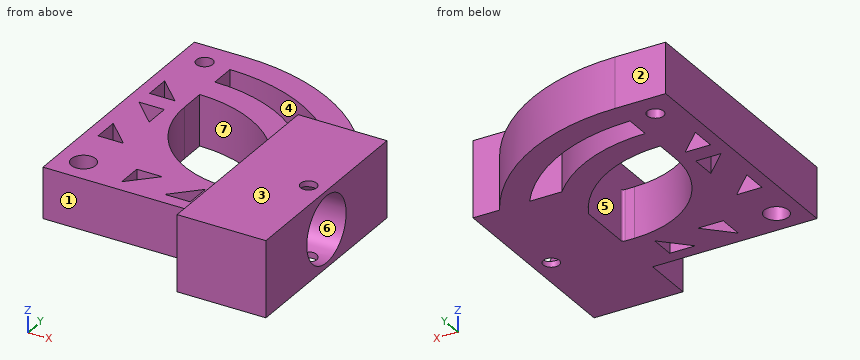
from build123d import *

# Parameters (mm, degrees)
F0_R     = 4.75
F1_DEPTH = 20
F2_DEPTH = 30
F3_R     = 13
F4_DEPTH = 25


with BuildPart() as f1:
    # F0 (on Top) → F1 (new body)
    with BuildSketch(Plane.XY):
        with BuildLine():
            Line((76.6160202911, 30.1966461055), (66.1766930438, 30.1966461055))
            ThreePointArc((66.1766930438, 30.1966461055), (73.2373422542, 14.1088810364), (76.6160202911, -3.132159736))
            Line((76.6160202911, -3.132159736), (76.6160202911, 30.1966461055))
        make_face()
        with BuildLine():
            ThreePointArc((76.6160202911, -3.132159736), (73.2373422542, 14.1088810364), (66.1766930438, 30.1966461055))
            Line((66.1766930438, 30.1966461055), (54.3402872065, 30.1966461055))
            ThreePointArc((54.3402872065, 30.1966461055), (63.4377209443, 11.9226935784), (66.8762698088, -8.198862606))
            ThreePointArc((66.8762698088, -8.198862606), (70.4472594921, -6.7390976404), (72.7910202911, -9.8033538945))
            ThreePointArc((72.7910202911, -9.8033538945), (70.4472594921, -12.8676101486), (66.8762698088, -11.407845183))
            ThreePointArc((66.8762698088, -11.407845183), (63.4377209443, -31.5294013674), (54.3402872065, -49.8033538945))
            Line((54.3402872065, -49.8033538945), (66.1766930438, -49.8033538945))
            ThreePointArc((66.1766930438, -49.8033538945), (73.2373422542, -33.7155888254), (76.6160202911, -16.474548053))
            Line((76.6160202911, -16.474548053), (76.6160202911, -3.132159736))
        make_face()
        with BuildLine():
            ThreePointArc((66.8762698088, -8.198862606), (63.4377209443, 11.9226935784), (54.3402872065, 30.1966461055))
            Line((54.3402872065, 30.1966461055), (41.6160202911, 30.1966461055))
            ThreePointArc((41.6160202911, 30.1966461055), (52.9450022789, 11.6059714919), (56.8946607411, -9.8033538945))
            ThreePointArc((56.8946607411, -9.8033538945), (52.9450022789, -31.2126792809), (41.6160202911, -49.8033538945))
            Line((41.6160202911, -49.8033538945), (54.3402872065, -49.8033538945))
            ThreePointArc((54.3402872065, -49.8033538945), (63.4377209443, -31.5294013674), (66.8762698088, -11.407845183))
            ThreePointArc((66.8762698088, -11.407845183), (66.4410202911, -9.8033538945), (66.8762698088, -8.198862606))
        make_face()
        with BuildLine():
            ThreePointArc((76.6160202911, -16.474548053), (73.2373422542, -33.7155888254), (66.1766930438, -49.8033538945))
            Line((66.1766930438, -49.8033538945), (76.6160202911, -49.8033538945))
            Line((76.6160202911, -49.8033538945), (76.6160202911, -16.474548053))
        make_face()
        with BuildLine():
            ThreePointArc((56.8946607411, -9.8033538945), (52.9450022789, 11.6059714919), (41.6160202911, 30.1966461055))
            Line((41.6160202911, 30.1966461055), (41.6160202911, 12.5573258805))
            ThreePointArc((41.6160202911, 12.5573258805), (45.5571102145, 1.6842921329), (46.8946607411, -9.8033538945))
            ThreePointArc((46.8946607411, -9.8033538945), (45.5571102145, -21.2909999219), (41.6160202911, -32.1640336695))
            Line((41.6160202911, -32.1640336695), (41.6160202911, -49.8033538945))
            ThreePointArc((41.6160202911, -49.8033538945), (52.9450022789, -31.2126792809), (56.8946607411, -9.8033538945))
        make_face()
        with BuildLine():
            ThreePointArc((46.8946607411, -9.8033538945), (45.5571102145, 1.6842921329), (41.6160202911, 12.5573258805))
            Line((41.6160202911, 12.5573258805), (41.6160202911, -8.8033538945))
            Line((41.6160202911, -8.8033538945), (41.6160202911, -29.8033538945))
            Line((41.6160202911, -29.8033538945), (41.6160202911, -30.8033538945))
            Line((41.6160202911, -30.8033538945), (41.6160202911, -32.1640336695))
            ThreePointArc((41.6160202911, -32.1640336695), (45.5571102145, -21.2909999219), (46.8946607411, -9.8033538945))
        make_face()
        with BuildLine():
            Line((-3.1053392589, 30.1966461055), (-3.1053392589, 40.1966461055))
            ThreePointArc((-3.1053392589, 40.1966461055), (-8.9600600243, 39.8526854639), (-14.7342290493, 38.8255358959))
            Line((-14.7342290493, 38.8255358959), (-8.1053392589, 32.1966461055))
            Line((-8.1053392589, 32.1966461055), (-18.1053392589, 32.1966461055))
            Line((-18.1053392589, 32.1966461055), (-18.1053392589, 37.8936061763))
            ThreePointArc((-18.1053392589, 37.8936061763), (-20.630331421, 37.0247856128), (-23.1053392589, 36.0224030551))
            Line((-23.1053392589, 36.0224030551), (-23.1053392589, -29.8033538945))
            Line((-23.1053392589, -29.8033538945), (-3.1053392589, -29.8033538945))
            Line((-3.1053392589, -29.8033538945), (40.6160202911, -29.8033538945))
            Line((40.6160202911, -29.8033538945), (41.6160202911, -29.8033538945))
            Line((41.6160202911, -29.8033538945), (41.6160202911, -8.8033538945))
            ThreePointArc((41.6160202911, -8.8033538945), (41.3231270723, -9.5104606757), (40.6160202911, -9.8033538945))
            Line((40.6160202911, -9.8033538945), (36.8946607411, -9.8033538945))
            ThreePointArc((36.8946607411, -9.8033538945), (8.6103894936, 1.912374858), (-3.1053392589, 30.1966461055))
        make_face()
        with Locations((-13.1053392589, -19.8033538945)):
            Circle(F0_R, mode=Mode.SUBTRACT)
        Polygon((4.8946607411, -14.8033538945), (14.8946607411, -14.8033538945), (4.8946607411, -24.8033538945), align=None, mode=Mode.SUBTRACT)
        Polygon((31.8946607411, -24.8033538945), (21.8946607411, -24.8033538945), (31.8946607411, -14.8033538945), align=None, mode=Mode.SUBTRACT)
        Polygon((-18.1053392589, -1.8033538945), (-18.1053392589, 8.1966461055), (-8.1053392589, -1.8033538945), align=None, mode=Mode.SUBTRACT)
        Polygon((-8.1053392589, 25.1966461055), (-8.1053392589, 15.1966461055), (-18.1053392589, 25.1966461055), align=None, mode=Mode.SUBTRACT)
        with BuildLine():
            Line((-3.1053392589, 40.1966461055), (-3.1053392589, 50.1966461055))
            ThreePointArc((-3.1053392589, 50.1966461055), (-13.2514579825, 49.3325596847), (-23.1053392589, 46.7651886004))
            Line((-23.1053392589, 46.7651886004), (-23.1053392589, 36.0224030551))
            ThreePointArc((-23.1053392589, 36.0224030551), (-20.630331421, 37.0247856128), (-18.1053392589, 37.8936061763))
            Line((-18.1053392589, 37.8936061763), (-18.1053392589, 42.1966461055))
            Line((-18.1053392589, 42.1966461055), (-14.7342290493, 38.8255358959))
            ThreePointArc((-14.7342290493, 38.8255358959), (-8.9600600243, 39.8526854639), (-3.1053392589, 40.1966461055))
        make_face()
        with BuildLine():
            Line((-3.1053392589, 50.1966461055), (-3.1053392589, 60.1966461055))
            ThreePointArc((-3.1053392589, 60.1966461055), (-6.4925947199, 60.1146445068), (-9.8719141705, 59.8688318324))
            ThreePointArc((-9.8719141705, 59.8688318324), (-12.6457198511, 56.9793102511), (-16.1176393473, 58.9765853786))
            ThreePointArc((-16.1176393473, 58.9765853786), (-19.6333066276, 58.2174245093), (-23.1053392589, 57.2786854305))
            Line((-23.1053392589, 57.2786854305), (-23.1053392589, 46.7651886004))
            ThreePointArc((-23.1053392589, 46.7651886004), (-13.2514579825, 49.3325596847), (-3.1053392589, 50.1966461055))
        make_face()
        with BuildLine():
            Line((-3.1053392589, 60.1966461055), (-3.1053392589, 70.1966461055))
            ThreePointArc((-3.1053392589, 70.1966461055), (-13.1856826575, 69.5590218069), (-23.1053392589, 67.6563130296))
            Line((-23.1053392589, 67.6563130296), (-23.1053392589, 57.2786854305))
            ThreePointArc((-23.1053392589, 57.2786854305), (-19.6333066276, 58.2174245093), (-16.1176393473, 58.9765853786))
            ThreePointArc((-16.1176393473, 58.9765853786), (-13.7268393445, 63.3866676797), (-9.8553392589, 60.1966461055))
            ThreePointArc((-9.8553392589, 60.1966461055), (-9.8594856318, 60.0325295879), (-9.8719141705, 59.8688318324))
            ThreePointArc((-9.8719141705, 59.8688318324), (-6.4925947199, 60.1146445068), (-3.1053392589, 60.1966461055))
        make_face()
        with BuildLine():
            ThreePointArc((-23.1053392589, 67.6563130296), (-13.1856826575, 69.5590218069), (-3.1053392589, 70.1966461055))
            Line((-3.1053392589, 70.1966461055), (-23.1053392589, 70.1966461055))
            Line((-23.1053392589, 70.1966461055), (-23.1053392589, 67.6563130296))
        make_face()
        with BuildLine():
            ThreePointArc((66.1766930438, 30.1966461055), (36.8946607411, 59.4786784083), (-3.1053392589, 70.1966461055))
            Line((-3.1053392589, 70.1966461055), (-3.1053392589, 60.1966461055))
            ThreePointArc((-3.1053392589, 60.1966461055), (29.2983642331, 52.2450143355), (54.3402872065, 30.1966461055))
            Line((54.3402872065, 30.1966461055), (66.1766930438, 30.1966461055))
        make_face()
        with BuildLine():
            ThreePointArc((41.6160202911, 30.1966461055), (21.3895581689, 44.968901856), (-3.1053392589, 50.1966461055))
            Line((-3.1053392589, 50.1966461055), (-3.1053392589, 40.1966461055))
            ThreePointArc((-3.1053392589, 40.1966461055), (23.181216347, 32.7291865231), (41.6160202911, 12.5573258805))
            Line((41.6160202911, 12.5573258805), (41.6160202911, 30.1966461055))
        make_face()
    extrude(amount=F1_DEPTH)

    # F0 (on Top) → F2 (join)
    with BuildSketch(Plane.XY):
        with BuildLine():
            ThreePointArc((56.8946607411, -9.8033538945), (52.9450022789, 11.6059714919), (41.6160202911, 30.1966461055))
            Line((41.6160202911, 30.1966461055), (41.6160202911, 12.5573258805))
            ThreePointArc((41.6160202911, 12.5573258805), (45.5571102145, 1.6842921329), (46.8946607411, -9.8033538945))
            ThreePointArc((46.8946607411, -9.8033538945), (45.5571102145, -21.2909999219), (41.6160202911, -32.1640336695))
            Line((41.6160202911, -32.1640336695), (41.6160202911, -49.8033538945))
            ThreePointArc((41.6160202911, -49.8033538945), (52.9450022789, -31.2126792809), (56.8946607411, -9.8033538945))
        make_face()
        with BuildLine():
            ThreePointArc((66.8762698088, -8.198862606), (63.4377209443, 11.9226935784), (54.3402872065, 30.1966461055))
            Line((54.3402872065, 30.1966461055), (41.6160202911, 30.1966461055))
            ThreePointArc((41.6160202911, 30.1966461055), (52.9450022789, 11.6059714919), (56.8946607411, -9.8033538945))
            ThreePointArc((56.8946607411, -9.8033538945), (52.9450022789, -31.2126792809), (41.6160202911, -49.8033538945))
            Line((41.6160202911, -49.8033538945), (54.3402872065, -49.8033538945))
            ThreePointArc((54.3402872065, -49.8033538945), (63.4377209443, -31.5294013674), (66.8762698088, -11.407845183))
            ThreePointArc((66.8762698088, -11.407845183), (66.4410202911, -9.8033538945), (66.8762698088, -8.198862606))
        make_face()
        with BuildLine():
            ThreePointArc((76.6160202911, -3.132159736), (73.2373422542, 14.1088810364), (66.1766930438, 30.1966461055))
            Line((66.1766930438, 30.1966461055), (54.3402872065, 30.1966461055))
            ThreePointArc((54.3402872065, 30.1966461055), (63.4377209443, 11.9226935784), (66.8762698088, -8.198862606))
            ThreePointArc((66.8762698088, -8.198862606), (70.4472594921, -6.7390976404), (72.7910202911, -9.8033538945))
            ThreePointArc((72.7910202911, -9.8033538945), (70.4472594921, -12.8676101486), (66.8762698088, -11.407845183))
            ThreePointArc((66.8762698088, -11.407845183), (63.4377209443, -31.5294013674), (54.3402872065, -49.8033538945))
            Line((54.3402872065, -49.8033538945), (66.1766930438, -49.8033538945))
            ThreePointArc((66.1766930438, -49.8033538945), (73.2373422542, -33.7155888254), (76.6160202911, -16.474548053))
            Line((76.6160202911, -16.474548053), (76.6160202911, -3.132159736))
        make_face()
        with BuildLine():
            ThreePointArc((76.6160202911, -16.474548053), (73.2373422542, -33.7155888254), (66.1766930438, -49.8033538945))
            Line((66.1766930438, -49.8033538945), (76.6160202911, -49.8033538945))
            Line((76.6160202911, -49.8033538945), (76.6160202911, -16.474548053))
        make_face()
        with BuildLine():
            Line((76.6160202911, 30.1966461055), (66.1766930438, 30.1966461055))
            ThreePointArc((66.1766930438, 30.1966461055), (73.2373422542, 14.1088810364), (76.6160202911, -3.132159736))
            Line((76.6160202911, -3.132159736), (76.6160202911, 30.1966461055))
        make_face()
        with BuildLine():
            ThreePointArc((46.8946607411, -9.8033538945), (45.5571102145, 1.6842921329), (41.6160202911, 12.5573258805))
            Line((41.6160202911, 12.5573258805), (41.6160202911, -8.8033538945))
            Line((41.6160202911, -8.8033538945), (41.6160202911, -29.8033538945))
            Line((41.6160202911, -29.8033538945), (41.6160202911, -30.8033538945))
            Line((41.6160202911, -30.8033538945), (41.6160202911, -32.1640336695))
            ThreePointArc((41.6160202911, -32.1640336695), (45.5571102145, -21.2909999219), (46.8946607411, -9.8033538945))
        make_face()
    extrude(amount=F2_DEPTH)

    # F3 (on face) → F4 (cut)
    with BuildSketch(Plane.YZ.offset(76.6160202911)):
        with Locations((-9.8033538945, 15)):
            Circle(F3_R)
    extrude(amount=-F4_DEPTH, mode=Mode.SUBTRACT)


solid = f1.part
Model file for the job. Use its own axes, mm. Face numbers are marked on the shaded views. A direction names the side the tool comes from. Round coordinates to 2 decimals unless told otherwise and drop trailing zeros. Loops run counter-clockwise (first coordinate to the right, second up) from the corner with the lowest first, then second, coordinate; pieces in that order, holes last. Notation, with made-up numbers: (82.5, 37.5) - (120.5, 37.5) arc R13 cw to (120.5, 42.5) - close; hole circle Ø5 at (65.5, -16). An arc over 180 degrees is marked (long way). Write each question's results on one line, items separated by ' | '.
(1) Wall check: L1, parallel to X at y = -21.5, z = 10; L2, parallel to X at y = -17.5, z = 2.5; L3, parallel to Z at x = 27.5, y = 39. Give the ranges that are in metal, low to high.
Answer below:
L1: x = -23.11 to -17.54, -8.67 to 4.89, 8.2 to 25.2, 31.89 to 51.62 | L2: x = -23.11 to -17.26, -8.95 to 4.89, 12.2 to 29.2, 31.89 to 76.62 | L3: z = 0 to 20
(2) Saw through at C-C, the plane z = 26. List the corners of the cut face in (x, y), then the cut area to 3 significant figures.
Answer below:
outline: (41.62, -49.8) - (76.62, -49.8) - (76.62, -16.73) - (51.62, -16.73) - (51.62, -2.88) - (76.62, -2.88) - (76.62, 30.2) - (41.62, 30.2) - close | area: 2,450 mm^2
(3) Saw through at B-B, the plane y = 34. List the corners of the cut face in (x, z).
Answer below:
outline: (-23.11, 0) - (-18.11, 0) - (-18.11, 20) - (-23.11, 20) - close; (-9.91, 0) - (-3.11, 0) - (-3.11, 20) - (-9.91, 20) - close; (21, 0) - (37.9, 0) - (37.9, 20) - (21, 20) - close; (51.5, 0) - (63.84, 0) - (63.84, 20) - (51.5, 20) - close
(4) Saw through at D-D, the plane y = -27. List the corners of the cut face in (x, z), then the cut area to 3 significant figures.
Answer below:
outline: (-23.11, 0) - (76.62, 0) - (76.62, 30) - (41.62, 30) - (41.62, 20) - (-23.11, 20) - close | area: 2,340 mm^2
(5) Saw through at A-A, the plane x = 58. List the corners of the cut face in (y, z), then the cut area to 3 significant figures.
Answer below:
outline: (-49.8, 0) - (41.83, 0) - (41.83, 20) - (30.2, 20) - (30.2, 30) - (-49.8, 30) - close; hole circle Ø26 at (-9.8, 15) | area: 2,100 mm^2
(6) Mould opens along Y. For the marked faces 1, 2, 3 and 4 say: released by +Y, released by -Y, zero draft, split by the parting line, or undercut.
Answer below:
face 1: released by -Y | face 2: released by +Y | face 3: zero draft | face 4: undercut
(7) 3-axis set-ups, long thin cutter, end or side, ignore diameter. For the marked faces 5, 6 and 7: which of +Z, -Z, +X, -X, +Y, -Y reach the whole face in a straight line?
Answer below:
face 5: +Z | face 6: +X | face 7: +Z, -Z
(8) Pin check, flat tips, straight feed: pin 1 (3 mm diameter, centred on x = 26.5, z = 9.5, fed in from +Y); pin 2 (10 mm diameter, centred on x = -2.5, z = 15, fed in from -Y); pin 3 (5 mm diameter, centred on y = 36, z = 12, fed in from +X). Stop position of each tip, or through.
Answer below:
pin 1: stops at y = 65.1 | pin 2: stops at y = -29.8 | pin 3: stops at x = 64.16
